Build history of the part. All positions in model axes, mm. Face numbers are marked on the shaded views. Round coordinates to 2 decimals unless told otherwise and drop trailing zeros. Loops run counter-clockwise (first coordinate to the right, second up) from the corner with the lowest first, then second, coordinate; pieces in that order, holes last. Notation, with made-up numbers: M 24,12 L 54,12 A23 ccw 54,27 Z; hole C 13.25,-35.5 d6. An arc over 180 degrees is marked long. Use one line per item in the form item = value. Start each with the question number.
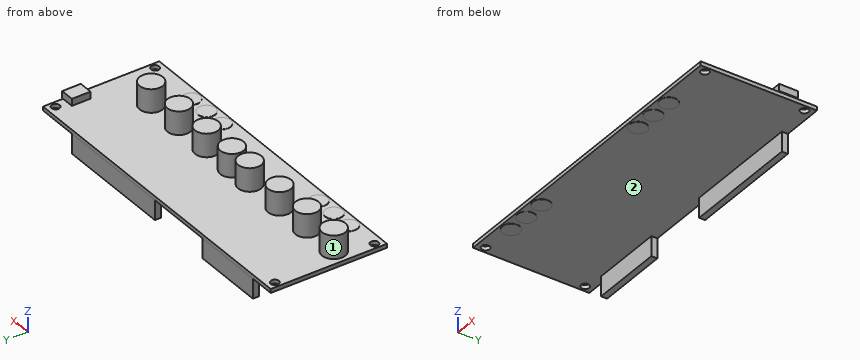
```python
from build123d import *

# Parameters (mm, degrees)
SKETCH1_W                = 140.5
SKETCH1_H                = 50
BOSS_EXTRUDE1_DEPTH      = 1.7
BOSS_EXTRUDE2_START      = 1.7
SKETCH1_3_R              = 5
BOSS_EXTRUDE2_DEPTH      = 10
BOSS_EXTRUDE3_START      = 1.7
SKETCH1_4_W              = 6
SKETCH1_4_H              = 8
BOSS_EXTRUDE3_DEPTH      = 3
SKETCH1_5_R              = 1.75
CUT_EXTRUDE1_DEPTH       = 76.943745628
SKETCH1_6_W              = 31
SKETCH1_6_H              = 2.59
SKETCH1_6_W_2            = 51
BOSS_EXTRUDE4_DEPTH      = 8.5
BOSS_EXTRUDE5_DEPTH      = 1.8
BOSS_EXTRUDE5_DEPTH_BACK = 0.1
SKETCH1_7_R              = 3.75


with BuildPart() as part:
    # Sketch1 → Boss-Extrude1 (new body)
    with BuildSketch(Plane.XY):
        Rectangle(SKETCH1_W, SKETCH1_H)
    extrude(amount=BOSS_EXTRUDE1_DEPTH)

    # Sketch1<3> → Boss-Extrude2 (add)
    with BuildSketch(Plane.XY.offset(BOSS_EXTRUDE2_START)):
        with Locations((-46.900113977, -6.9)):
            Circle(SKETCH1_3_R)
        with Locations((-63.386837135, -6.9)):
            Circle(SKETCH1_3_R)
        with Locations((-29.934803427, -6.9)):
            Circle(SKETCH1_3_R)
        with Locations((-11.533630076, -6.9)):
            Circle(SKETCH1_3_R)
        with Locations((-0.534156135, -6.9)):
            Circle(SKETCH1_3_R)
        with Locations((15.035822711, -6.9)):
            Circle(SKETCH1_3_R)
        with Locations((32.159770987, -6.9)):
            Circle(SKETCH1_3_R)
        with Locations((49.283975389, -6.9)):
            Circle(SKETCH1_3_R)
    extrude(amount=BOSS_EXTRUDE2_DEPTH)

    # Sketch1<4> → Boss-Extrude3 (add)
    with BuildSketch(Plane.XY.offset(BOSS_EXTRUDE3_START)):
        with Locations((67.75, 12.4)):
            Rectangle(SKETCH1_4_W, SKETCH1_4_H)
    extrude(amount=BOSS_EXTRUDE3_DEPTH)

    # Sketch1<5> → Cut-Extrude1 (cut, through all)
    with BuildSketch(Plane.XY):
        with Locations((-67.65, 21.4)):
            Circle(SKETCH1_5_R)
        with Locations(Location((67.65, 21.4, 0), (0, 0, 180))):
            Circle(SKETCH1_5_R)
        with Locations(Location((-67.65, -21.4, 0), (0, 0, 180))):
            Circle(SKETCH1_5_R)
        with Locations((67.65, -21.4)):
            Circle(SKETCH1_5_R)
    extrude(amount=CUT_EXTRUDE1_DEPTH, mode=Mode.SUBTRACT)

    # Sketch1<6> → Boss-Extrude4 (add)
    with BuildSketch(Plane.XY):
        with Locations((-43.75, 23.695)):
            Rectangle(SKETCH1_6_W, SKETCH1_6_H)
        with Locations((26.75, 23.695)):
            Rectangle(SKETCH1_6_W_2, SKETCH1_6_H)
    extrude(amount=-BOSS_EXTRUDE4_DEPTH)

    # Sketch1<7> → Boss-Extrude5 (add, two sides: drawn at the far end of the back side and taken through both)
    with BuildSketch(Plane.XY.offset(-BOSS_EXTRUDE5_DEPTH_BACK)):
        with Locations((-53.074008795, -20.6)):
            Circle(SKETCH1_7_R)
        with Locations((-43.706865007, -20.6)):
            Circle(SKETCH1_7_R)
        with Locations((-34.242336243, -20.6)):
            Circle(SKETCH1_7_R)
        with Locations((25.343402234, -20.6)):
            Circle(SKETCH1_7_R)
        with Locations((34.779018473, -20.6)):
            Circle(SKETCH1_7_R)
        with Locations((44.237672005, -20.6)):
            Circle(SKETCH1_7_R)
    extrude(amount=BOSS_EXTRUDE5_DEPTH + BOSS_EXTRUDE5_DEPTH_BACK)


solid = part.part
```
Q1. Wall check: probe 1 along Y at (x, z) = (67.65, 0.4); probe 2 along X at (y, z) = (21.4, 0.8); probe 3 along Z at (x, y) = (46, -15). Give the ranges that are in metal, low to high.
Q2. Drop flat-ended pins along their axis: P1, Ø1.5, axis at x = -43.5, y = 18, coming from the -Z side; P2, Ø8, axis at y = 0, z = -5, coming from the +X side; P3, Ø2, axis at x = 30.5, z = 8.5, coming from the -Y side; P4, Ø0.9, axis at y = 12.5, z = 3, coming from the -X side. Give the stop position or say it passes through.
Q3. Saw through at A-A (z = 6.75). Give the cut face in (x, y).
Q4. Pull direction Y, two halves, no side cores. Call the marked faces 1 and 2: pulls with the +Y half, pulls with the -Y half, needs draft (parallel to the pull), parting line crosses it, or undercut.
Q5. Saw through at B-B (x = 67.65). Give the cut face in (y, z).
Q6. Saw through at C-C (y = 11). Give the cut face in (x, z), and give its area (3 significant figures).
Q7. Saw through at D-D (z = -4.25). Give the cut face in (x, y), and give its area (3 significant figures).
Filled in:
q1.probe_1 = -25 to -23.15, -19.65 to 19.65, 23.15 to 25
q1.probe_2 = -70.25 to -69.4, -65.9 to 65.9, 69.4 to 70.25
q1.probe_3 = 0 to 1.7
q2.P1 = 0
q2.P2 = through
q2.P3 = -11.86
q2.P4 = 64.75
q3.outline = C -63.39,-6.9 d10; C -46.9,-6.9 d10; C -29.93,-6.9 d10; C -11.53,-6.9 d10; C -0.53,-6.9 d10; C 15.04,-6.9 d10; C 32.16,-6.9 d10; C 49.28,-6.9 d10
q4.face_1 = parting line crosses it
q4.face_2 = undercut
q5.outline = M -25,0 L -23.15,0 L -23.15,1.7 L -25,1.7 Z; M -19.65,0 L 19.65,0 L 19.65,1.7 L 16.4,1.7 L 16.4,4.7 L 8.4,4.7 L 8.4,1.7 L -19.65,1.7 Z; M 23.15,0 L 25,0 L 25,1.7 L 23.15,1.7 Z
q6.outline = M -70.25,0 L 70.25,0 L 70.25,1.7 L 70.75,1.7 L 70.75,4.7 L 64.75,4.7 L 64.75,1.7 L -70.25,1.7 Z
q6.area = 257 mm²
q7.outline = M -59.25,22.4 L -28.25,22.4 L -28.25,24.99 L -59.25,24.99 Z; M 1.25,22.4 L 52.25,22.4 L 52.25,24.99 L 1.25,24.99 Z
q7.area = 212 mm²
